Verification items for the finished model (mm, model axes). A direction names the side the tool comes from. Round coordinates to 2 decimals unless told otherwise and drop trailing zeros. Loops run counter-clockwise (first coordinate to the right, second up) from the corner with the lowest first, then second, coordinate; pieces in that order, holes last.
from build123d import *

# Parameters (mm, degrees)
BOSS_EXTRUDE1_DEPTH = 5.5
SKETCH2_W           = 15
SKETCH2_H           = 16.1125
BOSS_EXTRUDE2_DEPTH = 20
SKETCH3_W           = 6
SKETCH3_H           = 18
CUT_EXTRUDE1_DEPTH  = 6.5


with BuildPart() as part:
    # Sketch1 → Boss-Extrude1 (new body)
    with BuildSketch(Plane(origin=(0, 0, 0), x_dir=(1, 0, 0), z_dir=(0, 1, 0))):
        Polygon((0, 5.55625), (0, 8.05625), (15, 8.05625), (15, -8.05625), (0, -8.05625), (0, -5.55625), (3.207902433, -5.55625), (6.415804866, 0), (3.207902433, 5.55625), align=None)
    extrude(amount=BOSS_EXTRUDE1_DEPTH)

    # Sketch2 → Boss-Extrude2 (add)
    with BuildSketch(Plane(origin=(0, 5.5, 0), x_dir=(1, 0, 0), z_dir=(0, 1, 0))):
        with Locations((7.5, 0)):
            Rectangle(SKETCH2_W, SKETCH2_H)
    extrude(amount=BOSS_EXTRUDE2_DEPTH)

    # Sketch3 → Cut-Extrude1 (cut)
    with BuildSketch(Plane.ZY):
        with Locations((0, 16.5)):
            Rectangle(SKETCH3_W, SKETCH3_H)
    extrude(amount=-CUT_EXTRUDE1_DEPTH, mode=Mode.SUBTRACT)


solid = part.part
1. Tool access check on faces 1 (the face through (4.8, 2.7, 2.8)), 2 (the face through (3, 7.5, 0)), 3 (the face through (9, 0, 0)). Record the directions out of +Z, -Z, +X, -X, +Y, -Y that give a thin tool (end or side, any length) a straight path to the whole face; none if there is none.
2. Section check C-C (z = -5.25). Enter the section's corners in (x, y).
3. Section check A-A (y = 14.25). Enter the section's corners in (x, z).
4. Gauge pin test, flat ends, axial feed: P1, Ø1.9, axis at x = 2.5, z = -2.5, coming from the -Y side; P2, Ø1.8, axis at y = 19, z = 0.5, coming from the -X side; P3, Ø6, axis at x = 12, z = -2, coming from the -Y side. Record the tip position at first contact, or that the pin passes through.
5. Scan lines: L1, parallel to Z at x = 2, y = 23.5; L2, parallel to X at y = 23, z = -0.75; L3, parallel to Z at x = 1.75, y = 2.75. Record each from-to range of solid material in increasing order.
6. Section check B-B (x = 1). Enter the section's corners in (y, z), then the cut area to 3 significant figures.
7. Release check for a two-part mould opening along Z. For faces 4 (the face through (7, 13, -8.056)), 5 (the face through (7, 13, 8.056)), 6 (the face through (0, 13, 4)), 7 (the face through (3, 16, 3)) record: released by +Z, released by -Z, zero draft, split by the parting line, or undercut.
8. Section check D-D (y = 3.5). Enter the section's corners in (x, z).
Taken from the geometry:
1. face 1: -X, -Y
1. face 2: -X, +Y
1. face 3: +Z, -Z, +X, -X, -Y
2. outline: (0, 5.5) - (3.38, 5.5) - (3.38, 0) - (15, 0) - (15, 25.5) - (0, 25.5) - close
3. outline: (0, -8.06) - (15, -8.06) - (15, 8.06) - (0, 8.06) - (0, 3) - (6.5, 3) - (6.5, -3) - (0, -3) - close
4. P1: stops at y = 5.5
4. P2: stops at x = 6.5
4. P3: stops at y = 0
5. L1: z = -8.06 to -3, 3 to 8.06
5. L2: x = 6.5 to 15
5. L3: z = -8.06 to -5.56, 5.56 to 8.06
6. outline: (0, -8.06) - (25.5, -8.06) - (25.5, -3) - (7.5, -3) - (7.5, 3) - (25.5, 3) - (25.5, 8.06) - (0, 8.06) - (0, 5.56) - (5.5, 5.56) - (5.5, -5.56) - (0, -5.56) - close
6. area: 242 mm2
7. face 4: released by -Z
7. face 5: released by +Z
7. face 6: zero draft
7. face 7: undercut
8. outline: (0, -8.06) - (15, -8.06) - (15, 8.06) - (0, 8.06) - (0, 5.56) - (3.21, 5.56) - (6.42, 0) - (3.21, -5.56) - (0, -5.56) - close
